Design review of the part built by this model. Coordinates are the model's own, in mm. A direction names the side the tool comes from. Coordinates: 2 decimals unless noted, no trailing zeros. Use a Markdown table: item, result. Add a question column.
Q1. For faces 1 (the face through (616, 150.489, 173)), 2 (the face through (610, 153.308, 211)), 3 (the face through (-253, 3, 269)), list the 3-axis set-ups (+Z, -Z, +X, -X, +Y, -Y) from which the entire face can be reached by the end or side of a thin tool; tool diameter is ignored.
Q2. For probe 1 along Y at (x, z) = (-101, 148.5); probe 2 along Y at (x, z) = (651, 281), list the stretches that pass through material, from the lowest coordinate up.
Q3. Clearance check with flat-ended pins moving along their axes: pin 1 Ø1 at (x, z) = (-258, 235) entering from +Y; pin 2 Ø8 at (x, z) = (592.5, 174) entering from -Y; pin 3 Ø5 at (x, z) = (89.5, 75.5) entering from -Y. State where each tip first meets the part, or that it passes through.
from build123d import *

# Parameters (mm, degrees)
BOSS_EXTRUDE3_DEPTH = 350
SKETCH5_W           = 500
SKETCH5_H           = 30
BOSS_EXTRUDE4_DEPTH = 0.01
SKETCH6_W           = 438.972740408
SKETCH6_H           = 30
BOSS_EXTRUDE5_DEPTH = 0.01
SKETCH7_W           = 401.023798147
SKETCH7_H           = 30
BOSS_EXTRUDE6_DEPTH = 0.01


with BuildPart() as part:
    # Sketch2 → Boss-Extrude3 (new body)
    with BuildSketch(Plane.XY):
        Polygon((0, 0), (-500, 0), (-500, 3), (0, 3), (412.437530925, 153.307517797), (813.464753146, 153.307517797), (813.464753146, 150.488863063), (413.464753146, 150.488863063), align=None)
    extrude(amount=BOSS_EXTRUDE3_DEPTH)

    # Sketch5 → Boss-Extrude4 (add)
    with BuildSketch(Plane(origin=(0, 3, 0), x_dir=(1, 0, 0), z_dir=(0, 1, 0))):
        with Locations((-250, -175)):
            Rectangle(SKETCH5_W, SKETCH5_H)
    extrude(amount=BOSS_EXTRUDE4_DEPTH)

    # Sketch6 → Boss-Extrude5 (add)
    with BuildSketch(Plane(origin=(-0.965128259, 2.648271503, 0), x_dir=(0.9395515779432226, 0.34240740702327194, 0), z_dir=(-0.34240740702327194, 0.9395515779432226, 0))):
        with Locations((220.513592425, -175)):
            Rectangle(SKETCH6_W, SKETCH6_H)
    extrude(amount=BOSS_EXTRUDE5_DEPTH)

    # Sketch7 → Boss-Extrude6 (add)
    with BuildSketch(Plane(origin=(0, 153.307517797, 0), x_dir=(1, 0, 0), z_dir=(0, 1, 0))):
        with Locations((612.949429999, -175)):
            Rectangle(SKETCH7_W, SKETCH7_H)
    extrude(amount=BOSS_EXTRUDE6_DEPTH)


solid = part.part
Answer list:
| question | item | result |
|---|---|---|
| 1 | face 1 | +Z, -Z, +X, -Y |
| 1 | face 2 | +Z, -Z, +X, -X, +Y |
| 1 | face 3 | +Z, -Z, -X, +Y |
| 2 | probe 1 | 0 to 3 |
| 2 | probe 2 | 150.49 to 153.31 |
| 3 | pin 1 | y = 3 |
| 3 | pin 2 | y = 150.49 |
| 3 | pin 3 | y = 31.67 |
